Work out the finished part from the listing and answer in its coordinate system (mm). A direction names the side the tool comes from. Give positions to 0.01 mm unless a question says otherwise; leave off trailing zeros. Order: outer loops, then holes, each group sorted by start corner. A loop starts at its lowest first (then second) coordinate and runs counter-clockwise, first axis right, second up.
```python
from build123d import *

# Parameters (mm, degrees)
SKETCH1_W           = 93.6625
SKETCH1_H           = 40.64
SKETCH1_R           = 2.4892
BOSS_EXTRUDE1_DEPTH = 17.78
SKETCH6_R           = 3.96875
CUT_EXTRUDE4_DEPTH  = 104.635910312
CUT_EXTRUDE3_DEPTH  = 17.78
FILLET1_R           = 2.54
SKETCH3_R           = 4.064
CUT_EXTRUDE5_DEPTH  = 4.7752


with BuildPart() as part:
    # Sketch1 → Boss-Extrude1 (new body)
    with BuildSketch(Plane.XY):
        with Locations((-46.83125, 0)):
            Rectangle(SKETCH1_W, SKETCH1_H)
        with Locations((-84.93125, 0)):
            Circle(SKETCH1_R, mode=Mode.SUBTRACT)
        with Locations((-8.73125, 0)):
            Circle(SKETCH1_R, mode=Mode.SUBTRACT)
    extrude(amount=-BOSS_EXTRUDE1_DEPTH)

    # Sketch6 → Cut-Extrude4 (cut, through all)
    with BuildSketch(Plane(origin=(0, 20.32, 0), x_dir=(1, 0, 0), z_dir=(0, 1, 0))):
        with Locations(Location((-72.23125, 8.89, 0), (0, 0, 270))):
            Circle(SKETCH6_R)
        with Locations(Location((-21.43125, 8.89, 0), (0, 0, 270))):
            Circle(SKETCH6_R)
    extrude(amount=-CUT_EXTRUDE4_DEPTH, mode=Mode.SUBTRACT)

    # Sketch5 → Cut-Extrude3 (cut)
    with BuildSketch(Plane.XY):
        with BuildLine():
            Line((-93.6625, -20.32), (-93.6625, 20.32))
            Line((-93.6625, 20.32), (-84.93125, 20.32))
            Line((-84.93125, 20.32), (-84.93125, 10.622546022))
            ThreePointArc((-84.93125, 10.622546022), (-85.477262526, 9.049137635), (-86.880552326, 8.152186482))
            ThreePointArc((-86.880552326, 8.152186482), (-93.31325, 0), (-86.880552326, -8.152186482))
            ThreePointArc((-86.880552326, -8.152186482), (-85.477262526, -9.049137635), (-84.93125, -10.622546022))
            Line((-84.93125, -10.622546022), (-84.93125, -20.32))
            Line((-84.93125, -20.32), (-93.6625, -20.32))
        make_face()
        with BuildLine():
            Line((0, -20.32), (0, 20.32))
            Line((0, 20.32), (-8.73125, 20.32))
            Line((-8.73125, 20.32), (-8.73125, 10.622546022))
            ThreePointArc((-8.73125, 10.622546022), (-8.185237474, 9.049137635), (-6.781947674, 8.152186482))
            ThreePointArc((-6.781947674, 8.152186482), (-0.34925, 0), (-6.781947674, -8.152186482))
            ThreePointArc((-6.781947674, -8.152186482), (-8.185237474, -9.049137635), (-8.73125, -10.622546022))
            Line((-8.73125, -10.622546022), (-8.73125, -20.32))
            Line((-8.73125, -20.32), (0, -20.32))
        make_face()
    extrude(amount=-CUT_EXTRUDE3_DEPTH, mode=Mode.SUBTRACT)

    # Fillet1
    fillet1_edges = [part.edges().sort_by_distance(p)[0] for p in [
        (-84.93125, 20.32, -8.89),
        (-84.93125, -20.32, -8.89),
        (-8.73125, 20.32, -8.89),
        (-8.73125, -20.32, -8.89),
    ]]
    fillet(fillet1_edges, radius=FILLET1_R)

    # Sketch3 → Cut-Extrude5 (cut)
    with BuildSketch(Plane.XY):
        with Locations((-84.93125, 0)):
            Circle(SKETCH3_R)
        with Locations((-8.73125, 0)):
            Circle(SKETCH3_R)
    extrude(amount=-CUT_EXTRUDE5_DEPTH, mode=Mode.SUBTRACT)


solid = part.part
```
1. The part is cut by section D-D (y = -14.5). Write down the section's boundary in (x, z).
Findings below:
outline: (-84.93, -17.78) - (-8.73, -17.78) - (-8.73, 0) - (-84.93, 0) - close; hole circle Ø7.94 at (-72.23, -8.89); hole circle Ø7.94 at (-21.43, -8.89)
2. Straight lines are drawn through the part: probe 1 along X at (y, z) = (-10.5, -9); probe 2 along X at (y, z) = (-6, -11); probe 3 along Z at (x, y) = (-20, 6). For each, find the intervals that lie inside material, in ascending order.
Findings below:
probe 1: x = -84.93 to -76.2, -68.26 to -25.4, -17.46 to -8.73
probe 2: x = -90.78 to -75.59, -68.87 to -24.79, -18.07 to -2.88
probe 3: z = -17.78 to -12.59, -5.19 to 0
3. Which of the six approach directions +Z, -Z, +X, -X, +Y, -Y give full straight-line access (tool end or side, diameter ignored) to faces 1 (the face through (-84.931, 14, -9)), 2 (the face through (-8.731, -14, -9)), 3 (the face through (-83, 2, -4.775)), 4 (the face through (-84.167, -19.596, -9.014))?
Findings below:
face 1: +Z, -Z, -X, +Y
face 2: +Z, -Z, +X, -Y
face 3: +Z
face 4: +Z, -Z, -X, -Y
4. Given P1, Ø2, axis at y = 14.5, z = -12, coming from the -X side; P2, Ø2, axis at y = 13.5, z = -11, coming from the +X side; P3, Ø5, axis at y = -11, z = -4.5, coming from the +X side, each flat-ended and moving along its own axis, determine where each tip first touches the part or whether it passes through.
Findings below:
P1: stops at x = -84.93
P2: stops at x = -8.73
P3: stops at x = -7.59
5. The part is cut by section B-B (z = -15). Write down the section's boundary in (x, y).
Findings below:
outline: (-86.88, -8.15) arc R2.54 cw to (-84.93, -10.62) - (-84.93, -17.78) arc R2.54 ccw to (-82.39, -20.32) - (-11.27, -20.32) arc R2.54 ccw to (-8.73, -17.78) - (-8.73, -10.62) arc R2.54 cw to (-6.78, -8.15) arc R8.38 ccw to (-6.78, 8.15) arc R2.54 cw to (-8.73, 10.62) - (-8.73, 17.78) arc R2.54 ccw to (-11.27, 20.32) - (-82.39, 20.32) arc R2.54 ccw to (-84.93, 17.78) - (-84.93, 10.62) arc R2.54 cw to (-86.88, 8.15) arc R8.38 ccw to start; hole circle Ø4.98 at (-84.93, 0); hole circle Ø4.98 at (-8.73, 0)
6. The part is cut by section C-C (y = 0). Write down the section's boundary in (x, z), then the cut area to 3 significant figures.
Findings below:
outline: (-93.31, -17.78) - (-87.42, -17.78) - (-87.42, -4.78) - (-89, -4.78) - (-89, 0) - (-93.31, 0) - close; (-82.44, -17.78) - (-11.22, -17.78) - (-11.22, -4.78) - (-12.8, -4.78) - (-12.8, 0) - (-80.87, 0) - (-80.87, -4.78) - (-82.44, -4.78) - close; (-6.24, -17.78) - (-0.35, -17.78) - (-0.35, 0) - (-4.67, 0) - (-4.67, -4.78) - (-6.24, -4.78) - close; hole circle Ø7.94 at (-72.23, -8.89); hole circle Ø7.94 at (-21.43, -8.89)
area: 1,350 mm2
7. The part is cut by section A-A (z = -8.89). Write down the section's boundary in (x, y).
Findings below:
outline: (-86.88, -8.15) arc R2.54 cw to (-84.93, -10.62) - (-84.93, -17.78) arc R2.54 ccw to (-82.39, -20.32) - (-76.2, -20.32) - (-76.2, 20.32) - (-82.39, 20.32) arc R2.54 ccw to (-84.93, 17.78) - (-84.93, 10.62) arc R2.54 cw to (-86.88, 8.15) arc R8.38 ccw to start; (-68.26, -20.32) - (-25.4, -20.32) - (-25.4, 20.32) - (-68.26, 20.32) - close; (-17.46, -20.32) - (-11.27, -20.32) arc R2.54 ccw to (-8.73, -17.78) - (-8.73, -10.62) arc R2.54 cw to (-6.78, -8.15) arc R8.38 ccw to (-6.78, 8.15) arc R2.54 cw to (-8.73, 10.62) - (-8.73, 17.78) arc R2.54 ccw to (-11.27, 20.32) - (-17.46, 20.32) - close; hole circle Ø4.98 at (-84.93, 0); hole circle Ø4.98 at (-8.73, 0)
8. The mould has two halves that part along Y. Classify faces 5 (the face through (-85.46, 9.07, -8.77)), 6 (the face through (-8.731, 14, -9)), 7 (the face through (-11, -2, -4.775)): pulls with the +Y half, pulls with the -Y half, needs draft (parallel to the pull), parting line crosses it, or undercut.
Findings below:
face 5: pulls with the +Y half
face 6: needs draft
face 7: undercut
